```python
from build123d import *

# Parameters (mm, degrees)
SKETCH1_W                       = 26
SKETCH1_H                       = 51.5
EXTRUDE1_DEPTH                  = 5
SKETCH2_W                       = 18
SKETCH2_H                       = 28.3
EXTRUDE2_DEPTH                  = 5
FILLET1_R                       = 2.54
FILLET2_R                       = 18
EXTRUDE3_DEPTH                  = 26
SKETCH4_W                       = 26
SKETCH4_H                       = 5
EXTRUDE4_DEPTH                  = 1
F_4_40_TAPPED_HOLE1_D           = 2.2606
F_4_40_TAPPED_HOLE1_DEPTH       = 10.1346
F_4_40_TAPPED_HOLE1_CBORE_D     = 2.8448
F_4_40_TAPPED_HOLE1_CBORE_DEPTH = 8.2296
F_4_40_TAPPED_HOLE1_TIP         = 0.679152758
SKETCH6_R                       = 1.75
EXTRUDE5_DEPTH                  = 6.0000001
F_8_32_TAPPED_HOLE1_D           = 3.4544
F_8_32_TAPPED_HOLE1_DEPTH       = 10.7188
F_8_32_TAPPED_HOLE1_CBORE_D     = 4.1656
F_8_32_TAPPED_HOLE1_CBORE_DEPTH = 8.3312
F_8_32_TAPPED_HOLE1_TIP         = 1.037806461
F_4_40_TAPPED_HOLE2_D           = 2.2606
F_4_40_TAPPED_HOLE2_DEPTH       = 8.89
F_4_40_TAPPED_HOLE2_CBORE_D     = 2.8448
F_4_40_TAPPED_HOLE2_CBORE_DEPTH = 5.6896
F_4_40_TAPPED_HOLE2_TIP         = 0.679152758
SKETCH9_R                       = 0.5
EXTRUDE6_DEPTH                  = 2.032
BOSS_EXTRUDE2_DEPTH             = 26


with BuildPart() as part:
    # Sketch1 → Extrude1 (new body)
    with BuildSketch(Plane(origin=(0, 0, 0), x_dir=(1, 0, 0), z_dir=(0, 1, 0))):
        with Locations((-13, 25.75)):
            Rectangle(SKETCH1_W, SKETCH1_H)
    extrude(amount=EXTRUDE1_DEPTH)

    # Sketch2 → Extrude2 (cut)
    with BuildSketch(Plane(origin=(0, 5, 0), x_dir=(1, 0, 0), z_dir=(0, 1, 0))):
        with Locations((-9, 37.35)):
            Rectangle(SKETCH2_W, SKETCH2_H)
    extrude(amount=-EXTRUDE2_DEPTH, mode=Mode.SUBTRACT)

    # Fillet1
    fillet1_edges = [part.edges().sort_by_distance(p)[0] for p in [
        (0, 2.5, -23.2),
        (-18, 2.5, -51.5),
        (-26, 2.5, -51.5),
    ]]
    fillet(fillet1_edges, radius=FILLET1_R)

    # Fillet2
    fillet2_edges = [part.edges().sort_by_distance(p)[0] for p in [
        (-18, 2.5, -23.2),
    ]]
    fillet(fillet2_edges, radius=FILLET2_R)

    # Sketch3 → Extrude3 (add, through all)
    with BuildSketch(Plane(origin=(0, 0, 0), x_dir=(0, 0, -1), z_dir=(1, 0, 0))):
        Polygon((0, 5), (12.5, 5), (12.5, 10.7), (0.616783175, 9.029922788), (0.310602353, 11.20851254), (0, 11.164860226), align=None)
    extrude(amount=-EXTRUDE3_DEPTH)

    # Sketch4 → Extrude4 (cut)
    with BuildSketch(Plane.XY):
        with Locations((-13, 2.5)):
            Rectangle(SKETCH4_W, SKETCH4_H)
    extrude(amount=-EXTRUDE4_DEPTH, mode=Mode.SUBTRACT)

    # #4-40 Tapped Hole1
    with Locations(Plane(origin=(-22, 5, -48.2), x_dir=(0, 0, 1), z_dir=(0, 1, 0))):
        with Locations((0, 0)):
            CounterBoreHole(F_4_40_TAPPED_HOLE1_D / 2, F_4_40_TAPPED_HOLE1_CBORE_D / 2, F_4_40_TAPPED_HOLE1_CBORE_DEPTH, depth=F_4_40_TAPPED_HOLE1_DEPTH)
            with Locations((0, 0, -(F_4_40_TAPPED_HOLE1_DEPTH + F_4_40_TAPPED_HOLE1_TIP / 2))):  # 118° drill point
                Cone(0, F_4_40_TAPPED_HOLE1_D / 2, F_4_40_TAPPED_HOLE1_TIP, mode=Mode.SUBTRACT)

    # Sketch6 → Extrude5 (cut, through all)
    with BuildSketch(Plane(origin=(0, 5, 0), x_dir=(1, 0, 0), z_dir=(0, 1, 0))):
        with Locations(Location((-22, 41.2, 0), (0, 0, 270))):  # turned: the seam where the file's is
            Circle(SKETCH6_R)
    extrude(amount=-EXTRUDE5_DEPTH, mode=Mode.SUBTRACT)

    # #8-32 Tapped Hole1
    with Locations(Plane(origin=(-19.25, 9.864961394, -6.558391588), x_dir=(0, -0.139173101, 0.990268069), z_dir=(0, 0.990268069, 0.139173101))):
        with Locations((0, 0), (0, 12.5)):
            CounterBoreHole(F_8_32_TAPPED_HOLE1_D / 2, F_8_32_TAPPED_HOLE1_CBORE_D / 2, F_8_32_TAPPED_HOLE1_CBORE_DEPTH, depth=F_8_32_TAPPED_HOLE1_DEPTH)
            with Locations((0, 0, -(F_8_32_TAPPED_HOLE1_DEPTH + F_8_32_TAPPED_HOLE1_TIP / 2))):  # 118° drill point
                Cone(0, F_8_32_TAPPED_HOLE1_D / 2, F_8_32_TAPPED_HOLE1_TIP, mode=Mode.SUBTRACT)

    # #4-40 Tapped Hole2
    with Locations(Plane(origin=(-23, 2.5, -1), x_dir=(1, 0, 0), z_dir=(0, 0, 1))):
        with Locations((0, 0), (10, 0), (20, 0)):
            CounterBoreHole(F_4_40_TAPPED_HOLE2_D / 2, F_4_40_TAPPED_HOLE2_CBORE_D / 2, F_4_40_TAPPED_HOLE2_CBORE_DEPTH, depth=F_4_40_TAPPED_HOLE2_DEPTH)
            with Locations((0, 0, -(F_4_40_TAPPED_HOLE2_DEPTH + F_4_40_TAPPED_HOLE2_TIP / 2))):  # 118° drill point
                Cone(0, F_4_40_TAPPED_HOLE2_D / 2, F_4_40_TAPPED_HOLE2_TIP, mode=Mode.SUBTRACT)

    # Sketch9 → Extrude6 (cut)
    with BuildSketch(Plane.XZ):
        with Locations(Location((-23, -9.89, 0), (0, 0, 270))):  # turned: the seam where the file's is
            Circle(SKETCH9_R)
        with Locations(Location((-13, -9.89, 0), (0, 0, 270))):  # turned: the seam where the file's is
            Circle(SKETCH9_R)
        with Locations(Location((-3, -9.89, 0), (0, 0, 270))):  # turned: the seam where the file's is
            Circle(SKETCH9_R)
    extrude(amount=-EXTRUDE6_DEPTH, mode=Mode.SUBTRACT)

    # Sketch12 → Boss-Extrude2 (add)
    with BuildSketch(Plane(origin=(0, 0, 0), x_dir=(0, 0, -1), z_dir=(1, 0, 0))):
        Polygon((0, 11.164860226), (-0.5, 11.094589808), (-0.5, 5), (0, 5), align=None)
    extrude(amount=-BOSS_EXTRUDE2_DEPTH)


solid = part.part
```
Verification items for the finished model (mm, model axes). A direction names the side the tool comes from. Give positions to 0.01 mm unless a question says otherwise; leave off trailing zeros. Write each loop counter-clockwise with the first axis right and the second up, starting at its lowest first coordinate (ties: lowest second). Pieces come first, ordered by that corner, then holes. Notation, with made-up numbers: (73, 36) - (100, 36) arc R33 ccw to (100, 75) - close; hole circle Ø9 at (37.25, 10.25). An arc over 180 degrees is marked (long way). Put each result on its own line as item: value.
Q1. Section check B-B on z = -2.5. Record the cut outline in (x, y).
Result:
outline: (-26, 0) - (0, 0) - (0, 9.29) - (-26, 9.29) - close; hole circle Ø2.84 at (-23, 2.5); hole circle Ø2.84 at (-13, 2.5); hole circle Ø2.84 at (-3, 2.5)
Q2. Depth check by flat-ended pin: P1, Ø3, axis at x = -23, y = 3, coming from the +Z side; P2, Ø3, axis at x = -18.5, z = -40.5, coming from the +Y side; P3, Ø1.7, axis at x = -3, y = 2.5, coming from the -Z side; P4, Ø4, axis at x = -11, y = 3.5, coming from the +Z side. Enter the tip coordinate at first touch or a pass-through.
Result:
P1: z = -1
P2: y = 5
P3: z = -23.46
P4: z = 0.5
Q3. Section check A-A on z = -48.2. Record the cut outline in (x, y).
Result:
outline: (-26, 0) - (-23.42, 0) - (-23.42, 5) - (-26, 5) - close; (-20.58, 0) - (-18, 0) - (-18, 5) - (-20.58, 5) - close
Q4. Mould release check, pull along Y, two halves, no side actions. Record for faces 4 (the face through (-13, 8, -12.5)), 5 (the face through (-13, 5, 0)), 6 (the face through (-8.783, 5.86, -7.577)): released by +Y, released by -Y, zero draft, split by the parting line, or undercut.
Result:
face 4: zero draft
face 5: released by -Y
face 6: undercut
Q5. Section check D-D on z = -15.5. Record the cut outline in (x, y).
Result:
outline: (-26, 0) - (0, 0) - (0, 5) - (-26, 5) - close
Q6. Set-up check for faces 1 (the face through (-18, 3, -45)), 2 (the face through (-12.818, 10.104, -0.466)), 3 (the face through (-23.19, 3.91, -3.8)): record each of +Z, -Z, +X, -X, +Y, -Y from which the full face is reachable in a straight line by a thin tool's end or side.
Result:
face 1: -Z, +X, +Y, -Y
face 2: +X, -X, +Y
face 3: +Z
Q7. Section check C-C on y = 6.5. Count the separate pieces of the cut face and the enclosed holes in it, and give its area (3 significant figures).
Result:
separate pieces: 1
enclosed holes: 2
area: 310 mm2
Q8. Scan lines: probe 1 along X at (y, z) = (2.5, -7.55); probe 2 along X at (y, z) = (2.3, -48.2); probe 3 along Z at (x, y) = (-23, 0.6). Record each from-to range of solid material in increasing order. Write a range as from..to.
Result:
probe 1: -26..-24.13, -21.87..-21.33, -17.17..-14.13, -11.87..-8.83, -4.67..-4.13, -1.87..0
probe 2: -26..-23.42, -20.58..-18
probe 3: -51.5..-49.21, -47.19..-42.64, -39.76..-10.39, -9.39..-1
